```python
from build123d import *

# Parameters (mm, degrees)
SKETCH_1_W               = 15
SKETCH_1_H               = 15
EXTRUDE_1_DEPTH          = 41
SKETCH_2_W               = 33
SKETCH_2_H               = 15
CUT_EXTRUDE_1_DEPTH      = 10.686952674
CUT_EXTRUDE_3_DEPTH      = 47.16275555
CUT_EXTRUDE_3_DEPTH_BACK = 47.16275555
SKETCH_3_R               = 1.5
CUT_EXTRUDE_4_DEPTH      = 47.16275555
FILLET_1_R               = 2
FILLET_2_R               = 2
FILLET_3_R               = 2
FILLET_4_R               = 2
FILLET_5_R               = 2
FILLET_6_R               = 2
FILLET_7_R               = 2


with BuildPart() as part:
    # 草图1 → 凸台-拉伸1 (new body)
    with BuildSketch(Plane.XY):
        with Locations((7.5, -7.5)):
            Rectangle(SKETCH_1_W, SKETCH_1_H)
    extrude(amount=EXTRUDE_1_DEPTH)

    # 草图2 → 切除-拉伸1 (cut)
    with BuildSketch(Plane(origin=(15, 0, 0), x_dir=(0, 0, -1), z_dir=(1, 0, 0))):
        with Locations((-20.5, -7.5)):
            Rectangle(SKETCH_2_W, SKETCH_2_H)
    extrude(amount=-CUT_EXTRUDE_1_DEPTH, mode=Mode.SUBTRACT)

    # 草图3 → 切除-拉伸3 (cut, two sides: drawn at the far end of the back side and taken through both)
    with BuildSketch(Plane.XY.offset(41).offset(-CUT_EXTRUDE_3_DEPTH_BACK)):
        with Locations((7, -3.629065036)):
            Circle(SKETCH_3_R)
        with Locations((7, -10.409065036)):
            Circle(SKETCH_3_R)
    extrude(amount=CUT_EXTRUDE_3_DEPTH + CUT_EXTRUDE_3_DEPTH_BACK, mode=Mode.SUBTRACT)

    # 草图4 → 切除-拉伸4 (cut, through all)
    with BuildSketch(Plane.ZY):
        with BuildLine():
            Line((16.1, -4.363439511), (24.89752721, -4.363439511))
            ThreePointArc((24.89752721, -4.363439511), (27.970585717, -7.436498018), (24.89752721, -10.509556524))
            Line((24.89752721, -10.509556524), (16.1, -10.509556524))
            ThreePointArc((16.1, -10.509556524), (13.026941494, -7.436498018), (16.1, -4.363439511))
        make_face()
    extrude(amount=-CUT_EXTRUDE_4_DEPTH, mode=Mode.SUBTRACT)

    # 圆角1
    fillet_1_edges = [part.edges().sort_by_distance(p)[0] for p in [
        (7.5, 0, 41),
    ]]
    fillet(fillet_1_edges, radius=FILLET_1_R)

    # 圆角2
    # the kernel refuses this fillet: 2 mm, written as the material it adds along each edge
    with BuildSketch(Plane(origin=(4.313047326, 0, 37), x_dir=(1, 0, 0), z_dir=(0, -1, 0))) as fillet_2_piece_1_section:
        with BuildLine():
            CenterArc((FILLET_2_R, -FILLET_2_R), FILLET_2_R, 90, 90)
            Line((0, -FILLET_2_R), (0, 0))
            Line((0, 0), (FILLET_2_R, 0))
        make_face()
    fillet_2_piece_1 = extrude(amount=15, mode=Mode.PRIVATE)
    fillet_2_piece_1 = fillet_2_piece_1 - Plane(origin=(7, -10.409065036, 36.539920903), x_dir=(1, 0, 0), z_dir=(0, 0, 1)) * Cylinder(1.5, 38, mode=Mode.PRIVATE)
    fillet_2_piece_1 = fillet_2_piece_1 - Plane(origin=(7, -3.629065036, 36.539920903), x_dir=(1, 0, 0), z_dir=(0, 0, 1)) * Cylinder(1.5, 38, mode=Mode.PRIVATE)
    add(fillet_2_piece_1)

    # 圆角3
    # the kernel refuses this fillet: 2 mm, written as the material it adds along each edge
    with BuildSketch(Plane(origin=(4.313047326, -15, 4), x_dir=(0, 0, 1), z_dir=(0, 1, 0))) as fillet_3_piece_1_section:
        with BuildLine():
            CenterArc((FILLET_3_R, FILLET_3_R), FILLET_3_R, 180, 90)
            Line((0, FILLET_3_R), (0, 0))
            Line((0, 0), (FILLET_3_R, 0))
        make_face()
    fillet_3_piece_1 = extrude(amount=15, mode=Mode.PRIVATE)
    fillet_3_piece_1 = fillet_3_piece_1 - Plane(origin=(7, -10.409065036, 4.460079004), x_dir=(1, 0, 0), z_dir=(0, 0, 1)) * Cylinder(1.5, 38, mode=Mode.PRIVATE)
    fillet_3_piece_1 = fillet_3_piece_1 - Plane(origin=(7, -3.629065036, 4.460079004), x_dir=(1, 0, 0), z_dir=(0, 0, 1)) * Cylinder(1.5, 38, mode=Mode.PRIVATE)
    add(fillet_3_piece_1)

    # 圆角4
    fillet_4_edges = [part.edges().sort_by_distance(p)[0] for p in [
        (7.5, -15, 41),
    ]]
    fillet(fillet_4_edges, radius=FILLET_4_R)

    # 圆角5
    fillet_5_edges = [part.edges().sort_by_distance(p)[0] for p in [
        (7.5, 0, 0),
    ]]
    fillet(fillet_5_edges, radius=FILLET_5_R)

    # 圆角6
    fillet_6_edges = [part.edges().sort_by_distance(p)[0] for p in [
        (7.5, -15, 0),
    ]]
    fillet(fillet_6_edges, radius=FILLET_6_R)

    # 圆角7
    fillet_7_edges = [part.edges().sort_by_distance(p)[0] for p in [
        (0, -15, 20.5),
        (0, -14.414213562, 40.414213562),
        (0, -7.5, 0),
        (0, -0.585786438, 0.585786438),
        (0, -14.414213562, 0.585786438),
        (0, 0, 20.5),
        (0, -7.5, 41),
        (0, -0.585786438, 40.414213562),
    ]]
    fillet(fillet_7_edges, radius=FILLET_7_R)


solid = part.part
```
Can you work these out from the model? Positions are in its coordinate system, mm. A direction names the side the tool comes from. Coordinates: 2 decimals unless noted, no trailing zeros. Write each loop counter-clockwise with the first axis right and the second up, starting at its lowest first coordinate (ties: lowest second). Pieces come first, ordered by that corner, then holes. Notation, with made-up numbers: M 34.25,-12.5 L 58.25,-12.5 A17 ccw 58.25,10.5 Z; hole C 87.25,34.5 d11. An arc over 180 degrees is marked long. Answer as CSV lines item,"result".
Item 1: On a 3-axis mill with a long thin cutter (end or side, diameter ignored), from which of +Z, -Z, +X, -X, +Y, -Y can I reach the whole of each face in a straight line? I mean faces 4 (the flat face through (15, -8, 2)), 5 (the cylindrical face through (2.126, -7.504, 13.028)), 6 (the cylindrical face through (4.914, -7.605, 4.57)). Say none if no direction works.
Geometry results:
face 4,"+Z, -Z, +X, +Y, -Y"
face 5,"+X, -X"
face 6,"+X, +Y, -Y"
Item 2: We'd pull the mould along Z, two halves only. Please class faces 1 (the flat face through (11, -8, 37)), 2 (the flat face through (8, -7, 41)), 3 (the flat face through (4, 0, 22)): +Z half, -Z half, draft (parallel to the pull), parting line (faces both ways), or undercut.
Geometry results:
face 1,"undercut"
face 2,"+Z half"
face 3,"draft"
Item 3: Imagine slicing it at B-B on y = -8.5. List the corners of the cut face in (x, z) for me.
Geometry results:
outline,"M 0,2 A2 ccw 2,0 L 15,0 L 15,4 L 6.31,4 A2 cw 4.31,6 L 4.31,13.22 L 0,13.22 Z; M 0,27.78 L 4.31,27.78 L 4.31,35 A2 cw 6.31,37 L 15,37 L 15,41 L 2,41 A2 ccw 0,39 Z"
Item 4: Imagine slicing it at A-A on x = 9.25. List the corners of the cut face in (y, z) for me, plus the area to 3 significant figures.
Geometry results:
outline,"M -15,2 A2 ccw -13,0 L -2,0 A2 ccw 0,2 L 0,4 L -15,4 Z; M -15,37 L 0,37 L 0,39 A2 ccw -2,41 L -13,41 A2 ccw -15,39 Z"
area,"117 mm2"
Item 5: Imagine slicing it at C-C on x = 7. List the corners of the cut face in (y, z) for me, plus the area to 3 significant figures.
Geometry results:
outline,"M -15,2 A2 ccw -13,0 L -11.91,0 L -11.91,4 L -15,4 Z; M -15,37 L -11.91,37 L -11.91,41 L -13,41 A2 ccw -15,39 Z; M -8.91,0 L -5.13,0 L -5.13,4 L -8.91,4 Z; M -8.91,37 L -5.13,37 L -5.13,41 L -8.91,41 Z; M -2.13,0 L -2,0 A2 ccw 0,2 L 0,4 L -2.13,4 Z; M -2.13,37 L 0,37 L 0,39 A2 ccw -2,41 L -2.13,41 Z"
area,"68.6 mm2"
Item 6: Please list where these lines run through material, in increasing order: line 1 along Z through (x, y) = (13.5, -9.25); line 2 along Y through (x, z) = (6.75, 37.5); line 3 along Y through (x, z) = (7, 2.4).
Geometry results:
line 1,"z = 0 to 4, 37 to 41"
line 2,"y = -15 to -11.89, -8.93 to -5.11, -2.15 to 0"
line 3,"y = -15 to -11.91, -8.91 to -5.13, -2.13 to 0"
Item 7: Imagine slicing it at D-D on z = 14.5. List the corners of the cut face in (x, y) for me, plus the area to 3 significant figures.
Geometry results:
outline,"M 0,-13 A2 ccw 2,-15 L 4.31,-15 L 4.31,-10.06 L 0,-10.06 Z; M 0,-4.81 L 4.31,-4.81 L 4.31,0 L 2,0 A2 ccw 0,-2 Z"
area,"40.3 mm2"
Item 8: I'm going to push flat-ended pins straight in: P1, Ø5, axis at x = 8.5, z = 15.5, coming from the -Y side; P2, Ø4, axis at x = 4.5, z = 20.5, coming from the +Y side; P3, Ø7.5, axis at y = -6.5, z = 25, coming from the +X side. Where does each tip first touch, or does it pass through?
Geometry results:
P1,"passes through"
P2,"stops at y = 0"
P3,"stops at x = 4.31"
